```python
from build123d import *

# Parameters (mm, degrees)
SKETCH_1_W                     = 40
SKETCH_1_H                     = 40
SKETCH_1_R                     = 14.6
EXTRUDE_1_DEPTH                = 45
SKETCH_6_W                     = 1
SKETCH_6_H                     = 22
CUT_EXTRUDE_1_DEPTH            = 54.935146241
M3X0_5_1_D                     = 2.5
HOLE_START                     = -21
HOLE_WIZARD_M3_2_OUTLINE_R     = 3.25
HOLE_WIZARD_M3_2_OUTLINE_R_2   = 1.25
HOLE_WIZARD_M3_2_DEPTH         = 18
HOLE_START_2                   = -3
HOLE_WIZARD_M3_2_2_OUTLINE_R   = 1.7
HOLE_WIZARD_M3_2_2_OUTLINE_R_2 = 1.25
HOLE_WIZARD_M3_2_2_DEPTH       = 2.5
HOLE_WIZARD_M4_1_D             = 4.5
HOLE_WIZARD_M4_1_CBORE_D       = 8
HOLE_WIZARD_M4_1_CBORE_DEPTH   = 4.5
CUT_EXTRUDE_2_REACH            = 65.443
CUT_EXTRUDE_2_END_RADIUS       = 14.6
SKETCH_10_W                    = 13.5
SKETCH_10_H                    = 35
CUT_EXTRUDE_3_DEPTH            = 54.935146365
FILLET_3_DEPTH                 = 45
FILLET_4_R                     = 5


with BuildPart() as part:
    # 草圖1 → 填料-伸長1 (new body)
    with BuildSketch(Plane.XY):
        with Locations((0, 2)):
            Rectangle(SKETCH_1_W, SKETCH_1_H)
        with Locations(Location((0, 0, 0), (0, 0, 180))):
            Circle(SKETCH_1_R, mode=Mode.SUBTRACT)
    extrude(amount=EXTRUDE_1_DEPTH)

    # 草圖6 → 除料-伸長1 (cut, through all)
    with BuildSketch(Plane.XY.offset(45)):
        with Locations((0, 11)):
            Rectangle(SKETCH_6_W, SKETCH_6_H)
    extrude(amount=-CUT_EXTRUDE_1_DEPTH, mode=Mode.SUBTRACT)

    # M3x0.5 螺紋孔1 (through all)
    with Locations(Plane.ZY.offset(20)):
        with Locations((40, 18.295717922)):
            Hole(M3X0_5_1_D / 2)

    # M3 凹頭蓋螺釘的柱孔2: read off the stored shape, not the designer's step
    # M3 凹頭蓋螺釘的柱孔2 outline → M3 凹頭蓋螺釘的柱孔2 (cut)
    with BuildSketch(Plane.YZ.offset(HOLE_START)):
        with Locations((18.295717922, 40)):
            Circle(HOLE_WIZARD_M3_2_OUTLINE_R)
        with Locations((18.295717922, 40)):
            Circle(HOLE_WIZARD_M3_2_OUTLINE_R_2, mode=Mode.SUBTRACT)
    extrude(amount=HOLE_WIZARD_M3_2_DEPTH, mode=Mode.SUBTRACT)

    # Hole Wizard M3 _2 2 outline → Hole Wizard M3 _2 2 (cut)
    with BuildSketch(Plane.YZ.offset(HOLE_START_2)):
        with Locations((18.295717922, 40)):
            Circle(HOLE_WIZARD_M3_2_2_OUTLINE_R)
        with Locations((18.295717922, 40)):
            Circle(HOLE_WIZARD_M3_2_2_OUTLINE_R_2, mode=Mode.SUBTRACT)
    extrude(amount=HOLE_WIZARD_M3_2_2_DEPTH, mode=Mode.SUBTRACT)

    # M4 凹頭蓋螺釘的柱孔1 (through all)
    with Locations(Plane.XY.offset(45)):
        with Locations((15, -13), (-15, -13)):
            CounterBoreHole(HOLE_WIZARD_M4_1_D / 2, HOLE_WIZARD_M4_1_CBORE_D / 2, HOLE_WIZARD_M4_1_CBORE_DEPTH)

    # 除料-伸長2: up to this cylinder (the profile starts outside it)
    cut_extrude_2_end = Plane(origin=(0, 0, 15.25905), z_dir=(0, 0, -1)) * Cylinder(CUT_EXTRUDE_2_END_RADIUS, 161.086, mode=Mode.PRIVATE)
    # 草圖9 → 除料-伸長2 (cut, up to the surface)
    with BuildSketch(Plane.XZ.offset(-22), mode=Mode.PRIVATE) as cut_extrude_2_sk1:
        with BuildLine():
            Line((-10, 0), (10, 0))
            Line((10, 0), (10, 22.5))
            ThreePointArc((10, 22.5), (0, 32.5), (-10, 22.5))
            Line((-10, 22.5), (-10, 0))
        make_face()
    cut_extrude_2_tool1 = extrude(cut_extrude_2_sk1.sketch, amount=CUT_EXTRUDE_2_REACH, mode=Mode.PRIVATE) - cut_extrude_2_end
    add(cut_extrude_2_tool1.solids().sort_by_distance((0, 22, 15.25905))[0], mode=Mode.SUBTRACT)

    # 草圖10 → 除料-伸長3 (cut, through all)
    with BuildSketch(Plane(origin=(0, 0, 0), x_dir=(1, 0, 0), z_dir=(0, 1, 0))):
        with Locations((0, -17.5)):
            Rectangle(SKETCH_10_W, SKETCH_10_H)
    extrude(amount=-CUT_EXTRUDE_3_DEPTH, mode=Mode.SUBTRACT)

    # 圓角3: read off the stored shape, not the designer's step
    # 圓角3 outline → 圓角3 (cut)
    with BuildSketch(Plane.XY):
        with BuildLine():
            Line((20, 2.006250977), (20, 22))
            Line((20, 22), (0.5, 22))
            ThreePointArc((0.5, 22), (14.317821063, 15.970491021), (20, 2.006250977))
        make_face()
        with BuildLine():
            Line((-20, 22), (-20, 2.006250977))
            ThreePointArc((-20, 2.006250977), (-14.317821063, 15.970491021), (-0.5, 22))
            Line((-0.5, 22), (-20, 22))
        make_face()
    extrude(amount=FILLET_3_DEPTH, mode=Mode.SUBTRACT)

    # 圓角4
    fillet_4_edges = [part.edges().sort_by_distance(p)[0] for p in [
        (20, -18, 22.5),
        (-20, -18, 22.5),
    ]]
    fillet(fillet_4_edges, radius=FILLET_4_R)


solid = part.part
```
Here's how the part is built. I have some questions about the finished solid (model axes, mm). A direction names the side the tool comes from. Give positions to 0.01 mm unless a question says otherwise; leave off trailing zeros. Order: outer loops, then holes, each group sorted by start corner. A loop starts at its lowest first (then second) coordinate and runs counter-clockwise, first axis right, second up. Notation, with made-up numbers: (-36, 88.5) -> (13, 88.5) arc R5 ccw to (13, 95.5) -> close; hole circle Ø8 at (-15.75, 67.5). An arc over 180 degrees is marked (long way). Use CSV: the item, a comma, the result in double quotes. Start each with the question number.
Item 1: On a 3-axis mill with a long thin cutter (end or side, diameter ignored), from which of +Z, -Z, +X, -X, +Y, -Y can I reach the whole of each face in a straight line? I mean faces 1 (the cylindrical face through (7.319, 16.398, 29.315)), 2 (the flat face through (-0.5, 18, 37)), 3 (the cylindrical face through (-19, -16, 23)), 4 (the flat face through (17, -15, 40.5)). Say none if no direction works.
Item 2: Suppose I cut it at B-B (x = -2). List the corners of the cut face in (y, z) for me.
Item 3: I'm going to push flat-ended pins straight in: P1, Ø5, axis at x = 15, y = -13, coming from the +Z side; P2, Ø2.5, axis at x = -1.5, y = -15.5, coming from the -Z side; P3, Ø1.5, axis at x = 4.5, z = 25, coming from the +Y side; P4, Ø8, axis at y = 17, z = 40.5, coming from the +X side. Where does each tip first touch, or does it pass through?
Item 4: Suppose I cut it at C-C (y = -2). List the corners of the cut face in (x, z) for me, and give its area (3 significant figures).
Item 5: Thinking about a two-plate mould opening in X: for faces 5 (the flat face through (-3, 20, 39)), 6 (the cylindrical face through (-17.146, -12.324, 19.966)), 7 (the cylindrical face through (18, -17, 23)), which applies, pulls with the +X half, pulls with the -X half, needs draft (parallel to the pull), parting line crosses it, or undercut?
Item 6: If I drill on probe 1 along X at (y, z) = (-0.5, 8); probe 2 along Y at (x, z) = (-1, 39); probe 3 along X at (y, z) = (-2.5, 26), over which ranges is the centre line in solid material (lowest first)? Write a range as [from, to].
Item 7: Suppose I cut it at D-D (y = 5). List the corners of the cut face in (x, z) for me, and give its area (3 significant figures).
Item 8: Suppose I cut it at A-A (z = 10). List the corners of the cut face in (x, y) for me, and give its area (3 significant figures).
Answer block:
1,face 1,"-Z, +Y"
1,face 2,"+Z, -Z, +Y"
1,face 3,"+Z, -Z, -X, -Y"
1,face 4,"+Z"
2,outline,"(-18, 35) -> (-14.46, 35) -> (-14.46, 45) -> (-18, 45) -> close; (14.46, 32.3) -> (21.91, 32.3) -> (21.91, 45) -> (14.46, 45) -> close; hole circle Ø3.4 at (18.3, 40)"
3,P1,"stops at z = 40.5"
3,P2,"stops at z = 35"
3,P3,"passes through"
3,P4,"stops at x = 16.71"
4,outline,"(-20, 0) -> (-14.46, 0) -> (-14.46, 45) -> (-20, 45) -> close; (14.46, 0) -> (20, 0) -> (20, 45) -> (14.46, 45) -> close"
4,area,"498 mm^2"
5,face 5,"pulls with the -X half"
5,face 6,"undercut"
5,face 7,"pulls with the +X half"
6,probe 1,"x = [-20, -14.59], [14.59, 20]"
6,probe 2,"y = [-18, -14.57], [14.57, 16.92], [19.67, 21.98]"
6,probe 3,"x = [-20, -14.38], [14.38, 20]"
7,outline,"(-19.77, 0) -> (-13.72, 0) -> (-13.72, 45) -> (-19.77, 45) -> close; (13.72, 0) -> (19.77, 0) -> (19.77, 45) -> (13.72, 45) -> close"
7,area,"545 mm^2"
8,outline,"(-20, -13) arc R5 ccw to (-15, -18) -> (-6.75, -18) -> (-6.75, -12.95) arc R14.6 cw to (-10, 10.64) -> (-10, 19.33) arc R20 ccw to (-20, 2.01) -> close; (6.75, -18) -> (15, -18) arc R5 ccw to (20, -13) -> (20, 2.01) arc R20 ccw to (10, 19.33) -> (10, 10.64) arc R14.6 cw to (6.75, -12.95) -> close; hole circle Ø4.5 at (-15, -13); hole circle Ø4.5 at (15, -13)"
8,area,"508 mm^2"
